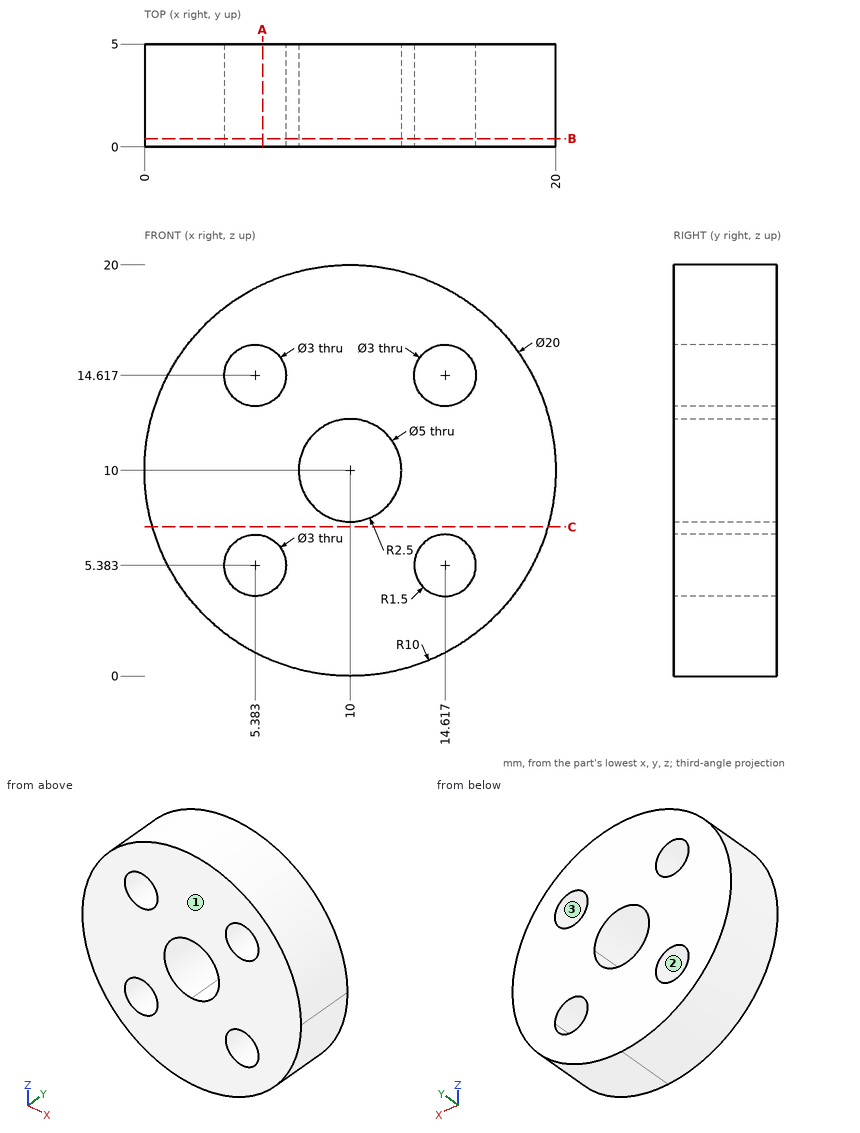
Print and shaded views of the part. All mm, measured from the part's lowest x, y and z. Coordinates: 2 decimals unless noted, no trailing zeros. Loops run counter-clockwise (first coordinate to the right, second up) from the corner with the lowest first, then second, coordinate; pieces in that order, holes last. Notation, with made-up numbers: (4.25, 82) -> (59.25, 82) arc R24 ccw to (59.25, 110) -> close; hole circle Ø5 at (-31.75, 36.25). An arc over 180 degrees is marked (long way). Use a Markdown table: item, result. Add a question column.
Item 1: Band-saw the part on A-A on x = 5.75. Write the cut outline in (y, z).
Item 2: Band-saw the part on C-C on z = 7.25. Write the cut outline in (x, y) (1 decimal).
Item 3: Flat gauge pins, fed straight in: P1, Ø1, axis at y = 1, z = 16, coming from the +X side; P2, Ø2, axis at y = 3.5, z = 11.5, coming from the -X side; P3, Ø2, axis at y = 3.5, z = 14.5, coming from the -X side. Where does each tip first touch, or does it go through?
Item 4: Band-saw the part on B-B on y = 0.4. Write the cut outline in (x, z), plus the area to 3 significant figures.
Item 5: Pull direction Z, two halves, no side cores. Call the marked faces 1, 2 and 3: +Z half, -Z half, draft (parallel to the pull), parting line (faces both ways), or undercut.
Item 6: Probe probe 1 along X at (y, z) = (1.25, 10); probe 2 along X at (y, z) = (3.9, 5.25) (1 decimal); probe 3 along Z at (x, y) = (6.5, 1) (1 decimal). List the from-to ranges inside material, lowest first.
Geometry says:
| question | item | result |
|---|---|---|
| 1 | outline | (0, 0.95) -> (5, 0.95) -> (5, 3.93) -> (0, 3.93) -> close; (0, 6.84) -> (5, 6.84) -> (5, 13.16) -> (0, 13.16) -> close; (0, 16.07) -> (5, 16.07) -> (5, 19.05) -> (0, 19.05) -> close |
| 2 | outline | (0.4, 0) -> (19.6, 0) -> (19.6, 5) -> (0.4, 5) -> close |
| 3 | P1 | x = 18.35 |
| 3 | P2 | x = 0.01 |
| 3 | P3 | x = 0.63 |
| 4 | outline | circle Ø20 at (10, 10); hole circle Ø3 at (5.38, 5.38); hole circle Ø3 at (5.38, 14.62); hole circle Ø5 at (10, 10); hole circle Ø3 at (14.62, 5.38); hole circle Ø3 at (14.62, 14.62) |
| 4 | area | 266 mm² |
| 5 | face 1 | draft |
| 5 | face 2 | undercut |
| 5 | face 3 | undercut |
| 6 | probe 1 | 0 to 7.5, 12.5 to 20 |
| 6 | probe 2 | 1.2 to 3.9, 6.9 to 13.1, 16.1 to 18.8 |
| 6 | probe 3 | 0.6 to 4.4, 6.4 to 13.6, 15.6 to 19.4 |
